Check sheet for the modelled part. Datum: model origin and axes. Units: mm. A direction names the side the tool comes from. Coordinates: 2 decimals unless noted, no trailing zeros. Loops run counter-clockwise (first coordinate to the right, second up) from the corner with the lowest first, then second, coordinate; pieces in that order, holes last. Notation, with made-up numbers: M 31.25,-5.5 L 78.25,-5.5 A18 cw 78.25,12.5 Z; hole C 42.25,34 d10. An arc over 180 degrees is marked long. Answer as CSV lines item,"result". Start each with the question number.
from build123d import *

# Parameters (mm, degrees)
F0_R          = 25
F0_R_2        = 2.5
F1_DEPTH      = 120
F2_DEPTH      = 30
F3_SIZE       = 2.5
F4_R          = 6.35
F5_DEPTH      = 25.001
F5_DEPTH_BACK = 25


with BuildPart() as f1:
    # F0 (on Top) → F1 (new body)
    with BuildSketch(Plane.XY):
        Circle(F0_R)
        Circle(F0_R_2, mode=Mode.SUBTRACT)
        Circle(F0_R_2)
    extrude(amount=F1_DEPTH)

    # F0 (on Top) → F2 (cut)
    with BuildSketch(Plane.XY):
        Circle(F0_R_2)
    extrude(amount=F2_DEPTH, mode=Mode.SUBTRACT)

    # F3
    f3_edges = [f1.edges().sort_by_distance(p)[0] for p in [
        (-2.5, 0, 30),
    ]]
    chamfer(f3_edges, length=F3_SIZE)

    # F4 (on Front) → F5 (cut, two sides)
    with BuildSketch(Plane.XZ) as f5_sk:
        with Locations((0, 105)):
            Circle(F4_R)
        with BuildLine():
            ThreePointArc((-30, 95), (0, 125), (30, 95))
            Line((30, 95), (51.988307, 95))
            Line((51.988307, 95), (51.988307, 154.9235))
            Line((51.988307, 154.9235), (-49.441047, 154.9235))
            Line((-49.441047, 154.9235), (-49.441047, 95))
            Line((-49.441047, 95), (-30, 95))
        make_face()
    extrude(amount=F5_DEPTH, mode=Mode.SUBTRACT)
    extrude(f5_sk.sketch, amount=-F5_DEPTH_BACK, mode=Mode.SUBTRACT)


solid = f1.part
Item 1: Sectioned sample at B-B, the plane z = 105. Record the boundary of the cut face in (x, y), and give its area (3 significant figures).
Item 2: Release check for a two-part mould opening along X. For faces 1 (the face through (-1.38, -0.36, 98.8)), 2 (the face through (0, 0, 120)), 3 (the face through (23.846, 7.509, 59.16)), 4 (the face through (20.19, 0.26, 117.19)) record: released by +X, released by -X, zero draft, split by the parting line, or undercut.
Item 3: Sectioned sample at D-D, the plane x = 21. Record the boundary of the cut face in (y, z), and give its area (3 significant figures).
Item 4: Material ranges on line 1 (Z direction, x = 0, y = 3); line 2 (X direction, y = 12, z = 105); line 3 (Z direction, x = 2.5, y = 10), recorded low to high. Write a range as from..to.
Item 5: Sectioned sample at C-C, the plane z = 63.5. Record the boundary of the cut face in (x, y), and give its area (3 significant figures).
Item 6: Go/stop test with flat-tipped pins: pin 1 (3 mm diameter, centred on x = -12, z = 97.5, fed in from +Y); pin 2 (8 mm diameter, centred on y = 6, z = 13.5, fed in from +X); pin 3 (1.5 mm diameter, centred on y = 12, z = 29.5, fed in from -X). Record where each tip stops, or that it passes through.
Item 7: Set-up check for faces 5 (the face through (-0.54, -2.44, 13.56)), 6 (the face through (-20.31, 0.26, 117.08)): record each of +Z, -Z, +X, -X, +Y, -Y from which the full face is reachable in a straight line by a thin tool's end or side.
Item 8: Sectioned sample at A-A, the plane y = -10.5. Record the boundary of the cut face in (x, z), and give its area (3 significant figures).
Reply:
1,outline,"M -6.35,-24.18 L -6.35,24.18 A25 ccw Z; M 6.35,-24.18 A25 ccw 6.35,24.18 Z"
1,area,"1,340 mm²"
2,face 1,"undercut"
2,face 2,"zero draft"
2,face 3,"split by the parting line"
2,face 4,"released by +X"
3,outline,"M -13.56,0 L 13.56,0 L 13.56,116.42 L -13.56,116.42 Z"
3,area,"3,160 mm²"
4,line 1,"0..98.65, 111.35..120"
4,line 2,"-21.93..-6.35, 6.35..21.93"
4,line 3,"0..99.16, 110.84..120"
5,outline,"C 0,0 d50"
5,area,"1,960 mm²"
6,pin 1,"y = 22.69"
6,pin 2,"x = 24.92"
6,pin 3,"x = -22.33"
7,face 5,"-Z"
7,face 6,"+Z, -X, +Y, -Y"
8,outline,"M -22.69,0 L 22.69,0 L 22.69,114.63 A30 ccw 16.58,120 L -16.58,120 A30 ccw -22.69,114.63 Z; hole C 0,105 d12.7"
8,area,"5,290 mm²"
